```python
from build123d import *

# Parameters (mm, degrees)
SKETCH1_W                                         = 69.85
SKETCH1_H                                         = 44.45
EXTRUDE1_DEPTH                                    = 4.7625
CBORE_FOR_1_4_PAN_HEAD_MACHINE_SCREW1_D           = 6.7564
CBORE_FOR_1_4_PAN_HEAD_MACHINE_SCREW1_CBORE_D     = 13.49248
CBORE_FOR_1_4_PAN_HEAD_MACHINE_SCREW1_CBORE_DEPTH = 4.445


with BuildPart() as part:
    # Sketch1 → Extrude1 (new body)
    with BuildSketch(Plane.XY):
        with Locations((0, 61.9125)):
            Rectangle(SKETCH1_W, SKETCH1_H)
    extrude(amount=EXTRUDE1_DEPTH)

    # CBORE for 1/4 Pan Head Machine Screw1 (through all)
    with Locations(Plane.XY.offset(4.7625)):
        with Locations((-19.05, 65.0875), (19.05, 65.0875)):
            CounterBoreHole(CBORE_FOR_1_4_PAN_HEAD_MACHINE_SCREW1_D / 2, CBORE_FOR_1_4_PAN_HEAD_MACHINE_SCREW1_CBORE_D / 2, CBORE_FOR_1_4_PAN_HEAD_MACHINE_SCREW1_CBORE_DEPTH)


solid = part.part
```
The listing builds one solid part. Answer for the finished solid, in the listing's coordinates (mm). A direction names the side the tool comes from. Coordinates: 2 decimals unless noted, no trailing zeros. Write each loop counter-clockwise with the first axis right and the second up, starting at its lowest first coordinate (ties: lowest second). Pieces come first, ordered by that corner, then holes. Notation, with made-up numbers: (54.25, 84) - (85.25, 84) arc R21 cw to (85.25, 101) - close; hole circle Ø5 at (-37.75, 12). An arc over 180 degrees is marked (long way). Return JSON: item names as keys, results as strings. Group by question number.
1. Which of the six approach directions +Z, -Z, +X, -X, +Y, -Y give full straight-line access (tool end or side, diameter ignored) to faces 1 (the cylindrical face through (19.49, 68.437, 0.157)), 2 (the cylindrical face through (-19.928, 71.776, 2.571))?
2. Straight lines are drawn through the part: L1, parallel to Y at x = -19.05, z = 3.6; L2, parallel to X at y = 68.5, z = 2.25 (1 decimal); L3, parallel to X at y = 70, z = 2.35 (3 decimals). For each, find the intervals that lie inside material, in ascending order.
3. Determine the mould class of faces 3 (the flat face through (0, 39.688, 2)), 4 (the cylindrical face through (-18.61, 68.437, 0.157)), 5 (the flat face through (-34.925, 62, 2)), 6 (the cylindrical face through (18.172, 71.776, 2.571)) for opening direction X: released by +X, released by -X, zero draft, split by the parting line, or undercut.
4. Given pin 1 (4 mm diameter, centred on x = 17.5, y = 65.5, fed in from +Z); pin 2 (5.5 mm diameter, centred on x = -19.05, y = 65.09, fed in from -Z), each flat-ended and moving along its own axis, determine where each tip first touches the part or whether it passes through.
5. A cutting plane is placed at A-A, the plane x = -19.05. Determine the outline of the cut face in (y, z), plus the area to 3 significant figures.
6. A cutting plane is placed at B-B, the plane y = 66. Give the number of separate pieces and of enclosed holes in the cut face, plus the area to 3 significant figures.
Ans:
{
 "1": {"face 1": "+Z, -Z", "face 2": "+Z"},
 "2": {"L1": "39.69 to 58.34, 71.83 to 84.14", "L2": "-34.9 to -24.9, -13.2 to 13.2, 24.9 to 34.9", "L3": "-34.925 to -23.674, -14.426 to 14.426, 23.674 to 34.925"},
 "3": {"face 3": "zero draft", "face 4": "undercut", "face 5": "released by -X", "face 6": "undercut"},
 "4": {"pin 1": "z = 0.32", "pin 2": "through"},
 "5": {"outline": "(39.69, 0) - (61.71, 0) - (61.71, 0.32) - (58.34, 0.32) - (58.34, 4.76) - (39.69, 4.76) - close; (68.47, 0) - (84.14, 0) - (84.14, 4.76) - (71.83, 4.76) - (71.83, 0.32) - (68.47, 0.32) - close", "area": "150 mm²"},
 "6": {"separate pieces": "3", "enclosed holes": "0", "area": "210 mm²"}
}
